```python
from build123d import *

# Parameters (mm, degrees)
F0_R     = 50
F1_DEPTH = 20
F2_R     = 19.99999
F3_R     = 45
F4_DEPTH = 10
F6_DEPTH = 25


# Not quite as in the source:
# - a fillet or chamfer is up to 0.001 mm smaller than in the source, because OpenCascade refuses the exact size


with BuildPart() as f1:
    # F0 (on Top) → F1 (new body)
    with BuildSketch(Plane.XY):
        Circle(F0_R)
    extrude(amount=F1_DEPTH)

    # F2 (radius 20 in the source; OpenCascade refuses exactly that, so slightly less here)
    f2_edges = [f1.edges().sort_by_distance(p)[0] for p in [
        (-50, 0, 20),
    ]]
    fillet(f2_edges, radius=F2_R)

    # F3 (on face) → F4 (cut)
    with BuildSketch(Plane(origin=(0, 0, 0), x_dir=(1, 0, 0), z_dir=(0, 0, -1))):
        Circle(F3_R)
    extrude(amount=-F4_DEPTH, mode=Mode.SUBTRACT)

    # F5 (on face) → F6 (cut)
    with BuildSketch(Plane.XY.offset(20)):
        with BuildLine():
            Line((-22.4775391325, -7.6695980696), (-44.9550782649, -15.3391961392))
            ThreePointArc((-44.9550782649, -15.3391961392), (-34.3172747897, -32.8416602961), (-17.2989432787, -44.2379538568))
            Line((-17.2989432787, -44.2379538568), (-8.6494716394, -22.1189769284))
            Line((-8.6494716394, -22.1189769284), (-22.4775391325, -7.6695980696))
        make_face()
        with BuildLine():
            Line((-7.6695980696, 22.4775391325), (-15.3391961392, 44.9550782649))
            ThreePointArc((-15.3391961392, 44.9550782649), (-32.8416602961, 34.3172747897), (-44.2379538568, 17.2989432787))
            Line((-44.2379538568, 17.2989432787), (-22.1189769284, 8.6494716394))
            Line((-22.1189769284, 8.6494716394), (-7.6695980696, 22.4775391325))
        make_face()
        with BuildLine():
            Line((22.4775391325, 7.6695980696), (44.9550782649, 15.3391961392))
            ThreePointArc((44.9550782649, 15.3391961392), (34.3172747897, 32.8416602961), (17.2989432787, 44.2379538568))
            Line((17.2989432787, 44.2379538568), (8.6494716394, 22.1189769284))
            Line((8.6494716394, 22.1189769284), (22.4775391325, 7.6695980696))
        make_face()
        with BuildLine():
            Line((7.6695980696, -22.4775391325), (15.3391961392, -44.9550782649))
            ThreePointArc((15.3391961392, -44.9550782649), (32.8416602961, -34.3172747897), (44.2379538568, -17.2989432787))
            Line((44.2379538568, -17.2989432787), (22.1189769284, -8.6494716394))
            Line((22.1189769284, -8.6494716394), (7.6695980696, -22.4775391325))
        make_face()
    extrude(amount=-F6_DEPTH, mode=Mode.SUBTRACT)


solid = f1.part
```
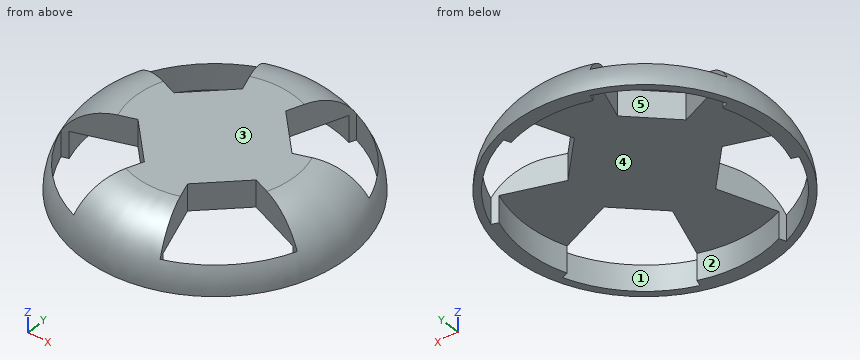
Design review of the part built by this model. Coordinates are the model's own, in mm. Face numbers are marked on the shaded views. A direction names the side the tool comes from. Give positions to 0.01 mm unless a question says otherwise; leave off trailing zeros. Loops run counter-clockwise (first coordinate to the right, second up) from the corner with the lowest first, then second, coordinate; pieces in that order, holes last. Notation, with made-up numbers: M 44.5,-5.5 L 68.5,-5.5 A23 cw 68.5,13.5 Z; hole C -11.75,74.25 d2. An arc over 180 degrees is marked long. Return JSON: item names as keys, results as strings. Group by question number.
Item 1: Insertion check: pin 1 Ø1 at (x, z) = (-11.5, 11) entering from +Y; pin 2 Ø10 at (y, z) = (-34.5, 16) entering from -X; pin 3 Ø5 at (y, z) = (29.5, 9) entering from -X. Each pin has a flat end and moves straight along its axis. Give the tip position at first contact, or say it passes through.
Item 2: We need section C-C (z = 8). Give the boundary of the cut face in (x, y), and give its area (3 significant figures).
Item 3: Tool access review of the marked faces 1 and 2: name each direction out of +Z, -Z, +X, -X, +Y, -Y from which nothing blocks a thin tool from reaching the whole face with its end or side.
Item 4: Mouldability with a two-part tool opening along X and no side actions: class the marked faces 3, 4 and 5 as released by +X, released by -X, zero draft, split by the parting line, or undercut.
Item 5: We need section D-D (y = -38.5). Give the number of separate pieces and of enclosed holes in the cut face, and give its area (3 significant figures).
Item 6: For probe 1 along Z at (x, y) = (13.5, 6.5); probe 2 along Y at (x, z) = (-18, 5); probe 3 along Y at (x, z) = (37, 1.5), list the stretches that pass through material, from the lowest coordinate up.
Output:
{
 "1": {"pin 1": "stops at y = 45.62", "pin 2": "stops at x = -15.44", "pin 3": "stops at x = -40"},
 "2": {"outline": "C 0,0 d96.66; hole M -44.96,-15.34 A47.5 ccw -17.3,-44.24 L -16.39,-41.91 A45 ccw 14.53,-42.59 L 15.34,-44.96 A47.5 ccw 44.24,-17.3 L 41.91,-16.39 A45 ccw 42.59,14.53 L 44.96,15.34 A47.5 ccw 17.3,44.24 L 16.39,41.91 A45 ccw -14.53,42.59 L -15.34,44.96 A47.5 ccw -44.24,17.3 L -41.91,16.39 A45 ccw -42.59,-14.53 Z", "area": "574 mm^2"},
 "3": {"face 1": "+Z, -Z", "face 2": "-Z"},
 "4": {"face 3": "zero draft", "face 4": "undercut", "face 5": "undercut"},
 "5": {"separate pieces": "3", "enclosed holes": "0", "area": "270 mm^2"},
 "6": {"probe 1": "z = 10 to 20", "probe 2": "y = -45.97 to -43.96, 43.96 to 45.97", "probe 3": "y = -33.55 to -29.79, 29.79 to 33.55"}
}
